Study the drawing (mm; zero at the part's minimum x, y, z) and answer. A direction names the side the tool comes from. Round coordinates to 2 decimals unless told otherwise and drop trailing zeros. Write each loop counter-clockwise with the first axis right and the second up, starting at its lowest first coordinate (ties: lowest second). Pieces come first, ordered by that corner, then holes.
(1) Each of these flat-tipped pins is pushed along its axis until it touches: pin 1 Ø4.5 at (x, z) = (4.28, 30.42) entering from +Y; pin 2 Ø2 at (x, z) = (34.59, 30.42) entering from +Y; pin 3 Ø6 at (x, y) = (34, 7) entering from -Z (1 decimal); pin 4 Ø5 at (x, y) = (5.5, 4) entering from -Z (1 decimal). Where does it stop, or does it pass through?
(2) A cutting plane is placed at B-B, the plane x = 18.5. Give the number of separate pieces and of enclosed holes in the cut face, and give its area (3 significant figures).
(3) For the marked faces 4 and 5, determine the directions among +Z, -Z, +X, -X, +Y, -Y from which every point of the face is accessible in a straight line to the end or side of a thin tool.
(4) Find the intervals of material crossed by probe 1 along X at (y, z) = (1.5, 30); probe 2 along Y at (x, z) = (31.5, 30); probe 3 along X at (y, z) = (2.25, 25.5) (1 decimal), in increasing order.
(5) A cutting plane is placed at C-C, the plane y = 7.5. Give the vertices of the cut face in (x, z) (1 decimal).
(6) A cutting plane is placed at D-D, the plane y = 12.75. Give the vertices of the cut face in (x, z).
(7) The mould has two halves that part along Z. Classify the marked faces 1, 2 and 3: +Z half, -Z half, draft (parallel to the pull), parting line (faces both ways), or undercut.
(8) A cutting plane is placed at A-A, the plane y = 3.5. Give the vertices of the cut face in (x, z), and give its area (3 significant figures).
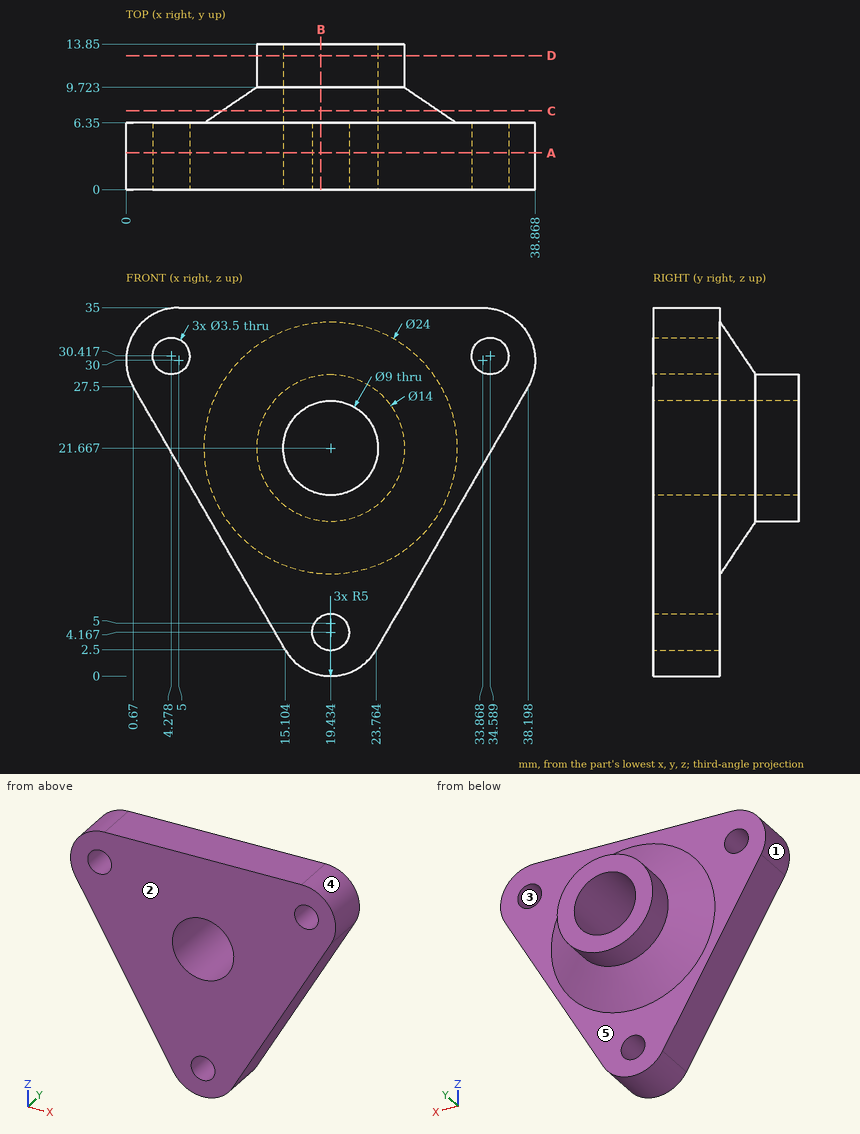
Solutions:
1. pin 1: stops at y = 6.35
1. pin 2: passes through
1. pin 3: stops at z = 15.2
1. pin 4: stops at z = 14.8
2. separate pieces: 3
2. enclosed holes: 0
2. area: 202 mm2
3. face 4: +X, +Y, -Y
3. face 5: +Y
4. probe 1: x = 0 to 2.58, 5.98 to 32.89, 36.29 to 38.87
4. probe 2: y = 0 to 6.35
4. probe 3: x = 1.8 to 17.1, 21.8 to 37
5. outline: circle Ø20.6 at (19.4, 21.7); hole circle Ø9 at (19.4, 21.7)
6. outline: circle Ø14 at (19.43, 21.67); hole circle Ø9 at (19.43, 21.67)
7. face 1: parting line
7. face 2: draft
7. face 3: undercut
8. outline: (0.67, 27.5) - (15.1, 2.5) arc R5 ccw to (23.76, 2.5) - (38.2, 27.5) arc R5 ccw to (33.87, 35) - (5, 35) arc R5 ccw to start; hole circle Ø3.5 at (4.28, 30.42); hole circle Ø9 at (19.43, 21.67); hole circle Ø3.5 at (19.43, 4.17); hole circle Ø3.5 at (34.59, 30.42)
8. area: 780 mm2
